Read the model definition and answer for the solid it produces. Units are mm, in the model's axes. A direction names the side the tool comes from. Coordinates: 2 decimals unless noted, no trailing zeros. Order: outer loops, then holes, each group sorted by start corner. A loop starts at its lowest first (then second) coordinate and runs counter-clockwise, first axis right, second up.
```python
from build123d import *

# Parameters (mm, degrees)
F0_R     = 12.7
F1_DEPTH = 139.7
F2_W     = 6.35
F2_H     = 31.75
F3_DEPTH = 30.734


with BuildPart() as f1:
    # F0 (on Top) → F1 (new body)
    with BuildSketch(Plane.XY):
        Circle(F0_R)
    extrude(amount=F1_DEPTH)

    # F2 (on Front) → F3 (cut)
    with BuildSketch(Plane.XZ):
        with Locations((0, 73.676325)):
            Rectangle(F2_W, F2_H)
    extrude(amount=-F3_DEPTH, mode=Mode.SUBTRACT)


solid = f1.part
```
1) A cutting plane is placed at D-D, the plane y = -3.5. Determine the outline of the cut face in (x, z), and give its area (3 significant figures).
A:
outline: (-12.21, 0) - (12.21, 0) - (12.21, 139.7) - (-12.21, 139.7) - close
area: 3,410 mm2
2) Which of the six approach directions +Z, -Z, +X, -X, +Y, -Y give full straight-line access (tool end or side, diameter ignored) to faces 1 (the flat face through (0, 0, 0)), 2 (the flat face through (0, 6, 57.801))?
A:
face 1: -Z, +X, -X, +Y, -Y
face 2: +Y
3) A cutting plane is placed at B-B, the plane y = 3. Determine the outline of the cut face in (x, z) (3 decimals).
A:
outline: (-12.341, 0) - (12.341, 0) - (12.341, 139.7) - (-12.341, 139.7) - close; hole (-3.175, 57.801) - (3.175, 57.801) - (3.175, 89.551) - (-3.175, 89.551) - close
4) A cutting plane is placed at C-C, the plane z = 62. Determine the outline of the cut face in (x, y) (3 decimals), and give its area (3 significant figures).
A:
outline: (-3.175, 0) - (-3.175, 12.297) arc R12.7 ccw (long way) to (3.175, 12.297) - (3.175, 0) - close
area: 427 mm2
5) Flat-ended cylindrical pins translate along their axes: pin 1 Ø1.5 at (x, z) = (4.5, 24) entering from +Y; pin 2 Ø8 at (x, z) = (-4.5, 33) entering from +Y; pin 3 Ø6 at (y, z) = (7, 75.5) entering from -X. Find the tip coordinate at first contact, or state that the pin passes through.
A:
pin 1: stops at y = 12.13
pin 2: stops at y = 12.69
pin 3: stops at x = -12.05
6) Straight lines are drawn through the part: line 1 (Z direction, x = -0.75, y = 6.5); line 2 (X direction, y = -0.5, z = 23.5); line 3 (X direction, y = 1, z = 75) (3 decimals). For each, find the intervals that lie inside material, in ascending order.
A:
line 1: z = 0 to 57.8, 89.55 to 139.7
line 2: x = -12.69 to 12.69
line 3: x = -12.661 to -3.175, 3.175 to 12.661
7) A cutting plane is placed at A-A, the plane x = 0. Determine the outline of the cut face in (y, z).
A:
outline: (-12.7, 0) - (12.7, 0) - (12.7, 57.8) - (0, 57.8) - (0, 89.55) - (12.7, 89.55) - (12.7, 139.7) - (-12.7, 139.7) - close
8) Determine the mould class of faces 3 (the flat face through (3.175, 6, 73)), 4 (the cylindrical face through (-2.75, -12.4, 68.87)), 5 (the flat face through (0, 0, 139.7)) for opening direction X: pulls with the +X half, pulls with the -X half, needs draft (parallel to the pull), parting line crosses it, or undercut.
A:
face 3: undercut
face 4: parting line crosses it
face 5: needs draft
